from build123d import *

# Parameters (mm, degrees)
SKETCH_2_W          = 170
SKETCH_2_H          = 170
EXTRUDE_1_DEPTH     = 140
SKETCH_3_W          = 150
SKETCH_3_H          = 150
CUT_EXTRUDE_1_DEPTH = 90
CUT_EXTRUDE_2_REACH = 152.167
SKETCH_4_W          = 80
SKETCH_4_H          = 75


with BuildPart() as part:
    # Эскиз2 → Бобышка-Вытянуть1 (new body)
    with BuildSketch(Plane(origin=(0, 0, 0), x_dir=(1, 0, 0), z_dir=(0, 1, 0))):
        Rectangle(SKETCH_2_W, SKETCH_2_H)
    extrude(amount=EXTRUDE_1_DEPTH)

    # Эскиз3 → Вырез-Вытянуть1 (cut)
    with BuildSketch(Plane(origin=(0, 140, 0), x_dir=(1, 0, 0), z_dir=(0, 1, 0))):
        Rectangle(SKETCH_3_W, SKETCH_3_H)
    extrude(amount=-CUT_EXTRUDE_1_DEPTH, mode=Mode.SUBTRACT)

    # Эскиз4 → Вырез-Вытянуть2 (cut, up to next)
    with BuildSketch(Plane(origin=(0, 50, 0), x_dir=(1, 0, 0), z_dir=(0, 1, 0)), mode=Mode.PRIVATE) as cut_extrude_2_sk1:
        Rectangle(SKETCH_4_W, SKETCH_4_H)
    cut_extrude_2_tool1 = extrude(cut_extrude_2_sk1.sketch, amount=-CUT_EXTRUDE_2_REACH, mode=Mode.PRIVATE) & part.part
    add(cut_extrude_2_tool1.solids().sort_by_distance((0, 50, 0))[0], mode=Mode.SUBTRACT)


solid = part.part
Verification items for the finished model (mm, model axes). A direction names the side the tool comes from. Coordinates: 2 decimals unless noted, no trailing zeros. Write each loop counter-clockwise with the first axis right and the second up, starting at its lowest first coordinate (ties: lowest second). Pieces come first, ordered by that corner, then holes. Notation, with made-up numbers: (-38.75, 28) - (15.25, 28) arc R32 cw to (15.25, 56) - close; hole circle Ø4 at (52, 73). An arc over 180 degrees is marked (long way). Answer as a JSON object with one key per item and string values.
(1) Gauge pin test, flat end, axial feed: pin 1 Ø2 at (x, z) = (64, 25) entering from +Y. Record the tip position at first contact, or that the pin passes through.
Report:
{"pin 1": "y = 50"}
(2) Thickness scan on line 1 along Z through (x, y) = (-61, 76); line 2 along Z through (x, y) = (-14.5, 40). Record the ranges inside material, lowest first.
Report:
{"line 1": "-85 to -75, 75 to 85", "line 2": "-85 to -37.5, 37.5 to 85"}
(3) Mould release check, pull along Z, two halves, no side actions. Record for faces 1 (the flat face through (-1, 69, -85)), 2 (the flat face through (-76, 140, 0)), 3 (the flat face through (-1, 50, 49)), 4 (the flat face through (-1, 69, 85)): pulls with the +Z half, pulls with the -Z half, needs draft (parallel to the pull), parting line crosses it, or undercut.
Report:
{"face 1": "pulls with the -Z half", "face 2": "needs draft", "face 3": "undercut", "face 4": "pulls with the +Z half"}
(4) Cross-section at A-A on x = -23. Record the cut outline in (y, z), plus the area to 3 significant figures.
Report:
{"outline": "(0, -85) - (140, -85) - (140, -75) - (50, -75) - (50, -37.5) - (0, -37.5) - close; (0, 37.5) - (50, 37.5) - (50, 75) - (140, 75) - (140, 85) - (0, 85) - close", "area": "6,550 mm^2"}
(5) Cross-section at D-D on z = 48.5. Record the cut outline in (x, y).
Report:
{"outline": "(-85, 0) - (85, 0) - (85, 140) - (75, 140) - (75, 50) - (-75, 50) - (-75, 140) - (-85, 140) - close"}
(6) Tool access check on faces 5 (the flat face through (-1, 0, -39)), 6 (the flat face through (75, 96, 1)), 7 (the flat face through (-1, 25, 37.5)). Record the directions out of +Z, -Z, +X, -X, +Y, -Y that give a thin tool (end or side, any length) a straight path to the whole face; none if there is none.
Report:
{"face 5": "+Z, -Z, +X, -X, -Y", "face 6": "+Y", "face 7": "+Y, -Y"}
(7) Cross-section at C-C on z = -32.5. Record the cut outline in (x, y), plus the area to 3 significant figures.
Report:
{"outline": "(-85, 0) - (-40, 0) - (-40, 50) - (-75, 50) - (-75, 140) - (-85, 140) - close; (40, 0) - (85, 0) - (85, 140) - (75, 140) - (75, 50) - (40, 50) - close", "area": "6,300 mm^2"}
(8) Cross-section at B-B on y = 84.5. Record the cut outline in (x, z), plus the area to 3 significant figures.
Report:
{"outline": "(-85, -85) - (85, -85) - (85, 85) - (-85, 85) - close; hole (-75, -75) - (75, -75) - (75, 75) - (-75, 75) - close", "area": "6,400 mm^2"}
